```python
from build123d import *

# Parameters (mm, degrees)
BOSS_EXTRUDE1_DEPTH = 14
CUT_EXTRUDE1_DEPTH  = 17
CUT_EXTRUDE3_DEPTH  = 10
CUT_EXTRUDE5_DEPTH  = 28.00000000000001
BOSS_EXTRUDE2_START = 10
SKETCH7_R           = 2.599999999999999
BOSS_EXTRUDE2_DEPTH = 4
BOSS_EXTRUDE3_DEPTH = 24.000000000000014
CUT_EXTRUDE6_DEPTH  = 24.000000000000014
FILLET3_R           = 10.371224
SKETCH11_R          = 2.0000000000000036
BOSS_EXTRUDE4_DEPTH = 4.0000000000000036
SKETCH12_R          = 5.999999999999998
CUT_EXTRUDE7_DEPTH  = 2
CUT_EXTRUDE8_START  = -2
SKETCH13_R          = 6.000000000000001
CUT_EXTRUDE8_DEPTH  = 2


with BuildPart() as part:
    # Sketch1 → Boss-Extrude1 (new body)
    with BuildSketch(Plane.XY):
        with BuildLine():
            Line((-36.38946679579018, 35.15986129833476), (18.20052051694879, -13.03747639081095))
            Line((18.20052051694879, -13.03747639081095), (35.77692020217122, -13.037476390810937))
            ThreePointArc((35.77692020217122, -13.037476390810937), (35.15777812721451, -10.159169225075718), (33.40987673348322, -7.79002807961883))
            Line((33.40987673348322, -7.79002807961883), (-19.19377778956647, 51.90227090989418))
            ThreePointArc((-19.19377778956647, 51.90227090989418), (-36.16282709845803, 52.12891060722632), (-36.38946679579018, 35.15986129833476))
        make_face()
    extrude(amount=BOSS_EXTRUDE1_DEPTH)

    # Sketch2 → Cut-Extrude1 (cut)
    with BuildSketch(Plane.XY.offset(14)):
        with BuildLine():
            ThreePointArc((-26.066464510259447, 45.48286358386564), (-29.74341977242946, 45.48286358386556), (-29.74341977242945, 41.80590832169555))
            Line((-29.74341977242943, 41.80590832169553), (-26.066464510259397, 45.48286358386558))
        make_face()
        with BuildLine():
            Line((-26.066464510259397, 45.48286358386558), (-29.74341977242943, 41.80590832169553))
            ThreePointArc((-29.74341977242945, 41.805908321695554), (-26.90996521719519, 41.24229916825121), (-25.304942141344416, 43.64438595278056))
            ThreePointArc((-25.304942141344416, 43.64438595278056), (-25.502855356815083, 44.63936287692983), (-26.066464510259447, 45.48286358386564))
        make_face()
    extrude(amount=-CUT_EXTRUDE1_DEPTH, mode=Mode.SUBTRACT)

    # Sketch3 → Cut-Extrude3 (cut)
    with BuildSketch(Plane(origin=(0, 0, 0), x_dir=(-1, 0, 0), z_dir=(0, 0, -1))):
        Polygon((9.244950076252596, 40.61278154184911), (25.60190789451236, 23.944622093291866), (43.70935849975749, 23.944622093291866), (43.70935849975749, 56.22709716223903), (9.244950076252595, 56.22709716223903), align=None)
    extrude(amount=-CUT_EXTRUDE3_DEPTH, mode=Mode.SUBTRACT)

    # Sketch4 → Cut-Extrude5 (cut)
    with BuildSketch(Plane(origin=(1.5041731974177077, 1.7036790764832412, 0), x_dir=(0.7496354730351515, -0.6618509330410925, 0), z_dir=(-0.6618509330410925, -0.7496354730351515, 0))):
        with BuildLine():
            Line((8.092649067523661, 8), (43.108918661974144, 8))
            Line((43.108918661974144, 8), (43.108918661974144, 14))
            Line((43.108918661974144, 14), (-35.75655339767276, 14))
            add(Edge.make_bspline(
                [(8.092649067523661, 8), (-13.064100153172822, 13.584073422401662), (-35.75655339767276, 14)],
                knots=[0, 0, 0, 1, 1, 1], degree=2))
        make_face()
    extrude(amount=-CUT_EXTRUDE5_DEPTH, mode=Mode.SUBTRACT)



with BuildPart() as body_2:
    # Sketch7 → Boss-Extrude2 (new body)
    with BuildSketch(Plane(origin=(0, 0, 10), x_dir=(-1, 0, 0), z_dir=(0, 0, -1)).offset(BOSS_EXTRUDE2_START)):
        with BuildLine():
            Line((9.244950076252595, 40.61278154184911), (24.71284152511152, 24.85060352151197))
            Line((24.71284152511152, 24.85060352151197), (35.272794661727836, 34.17395478721706))
            Line((35.272794661727836, 34.17395478721706), (36.38946679579018, 35.15986129833476))
            ThreePointArc((36.38946679579018, 35.15986129833476), (36.27690366691708, 52.016347478352856), (19.420417486898984, 52.12891060722668))
            ThreePointArc((19.420417486898984, 52.128910607226686), (19.259089791001077, 51.96445532507904), (19.10094915036315, 51.79693307859034))
            Line((19.10094915036315, 51.79693307859034), (18.710021655268264, 51.3533258590539))
            Line((18.710021655268264, 51.3533258590539), (9.244950076252596, 40.61278154184911))
        make_face()
        with Locations(Location((27.904942141344414, 43.64438595278056, 0), (0, 0, 180))):
            Circle(SKETCH7_R, mode=Mode.SUBTRACT)
    extrude(amount=BOSS_EXTRUDE2_DEPTH)


with BuildPart() as part_1:
    add(part.part)

    add(body_2.part)  # Boss-Extrude3 merges body 2
    # Sketch9 → Boss-Extrude3 (add)
    with BuildSketch(Plane(origin=(14.941459139681696, 13.167114819822281, 0), x_dir=(0, 0, -1), z_dir=(0.7502493779859964, 0.6611549522098625, 0))):
        with BuildLine():
            Line((0, 36.582058615900806), (0, -5.650867010397978))
            add(Edge.make_bspline(
                [(0, -5.650867010397978), (3.8818367436513204, 15.308651069653255), (4, 36.582058615900806)],
                knots=[0, 0, 0, 1, 1, 1], degree=2))
            Line((4, 36.582058615900806), (0, 36.582058615900806))
        make_face()
    extrude(amount=-BOSS_EXTRUDE3_DEPTH)

    # Sketch10 → Cut-Extrude6 (cut)
    with BuildSketch(Plane.XY):
        Polygon((-25.92087579699025, 25.91717339280068), (6.581343150758677, -2.7789391982650153), (-1.9207549102098282, -11.21281031813962), (-35.1442259060093, 19.61838673287275), align=None)
    extrude(amount=-CUT_EXTRUDE6_DEPTH, mode=Mode.SUBTRACT)

    # Fillet3
    fillet3_edges = [part_1.edges().sort_by_distance(p)[0] for p in [
        (-24.712841525111525, 24.85060352151197, 5),
        (-9.244950076252596, 40.61278154184911, 5),
    ]]
    fillet(fillet3_edges, radius=FILLET3_R - 0.0001)  # a hair under: the kernel refuses the full size

    # Sketch11 → Boss-Extrude4 (add)
    with BuildSketch(Plane.XY.offset(14)):
        with BuildLine():
            Line((-56.27002242528391, 53.500762526462196), (-36.38946679579018, 35.15986129833476))
            Line((-36.38946679579018, 35.15986129833476), (-31.30885180689802, 50.34187338631568))
            Line((-31.30885180689802, 50.34187338631568), (-18.71002165526834, 51.353325859054))
            Line((-18.71002165526834, 51.353325859054), (-40.42419503361445, 70.87498928012118))
            ThreePointArc((-40.42419503361445, 70.87498928012118), (-57.13470265149496, 73.54200286861439), (-59.89717634802535, 56.84701064326646))
            Line((-59.89717634802535, 56.84701064326646), (-56.27002242528391, 53.500762526462196))
        make_face()
        with Locations((-50.120598780049356, 63.8053531942874)):
            Circle(SKETCH11_R, mode=Mode.SUBTRACT)
    extrude(amount=-BOSS_EXTRUDE4_DEPTH)

    # Sketch12 → Cut-Extrude7 (cut)
    with BuildSketch(Plane(origin=(0, 0, -4), x_dir=(-1, 0, 0), z_dir=(0, 0, -1))):
        with Locations((27.904942141344414, 43.64438595278056)):
            Circle(SKETCH12_R)
    extrude(amount=-CUT_EXTRUDE7_DEPTH, mode=Mode.SUBTRACT)

    # Sketch13 → Cut-Extrude8 (cut)
    with BuildSketch(Plane.XY.offset(14).offset(CUT_EXTRUDE8_START)):
        with Locations(Location((-27.904942141344414, 43.64438595278056, 0), (0, 0, 180))):
            Circle(SKETCH13_R)
    extrude(amount=CUT_EXTRUDE8_DEPTH, mode=Mode.SUBTRACT)


solid = part_1.part
```
Can you work these out from the model? Positions are in its coordinate system, mm. A direction names the side the tool comes from. Coordinates: 2 decimals unless noted, no trailing zeros. Order: outer loops, then holes, each group sorted by start corner. A loop starts at its lowest first (then second) coordinate and runs counter-clockwise, first axis right, second up. Notation, with made-up numbers: (47.25, 89.25) -> (81.25, 89.25) arc R30 cw to (81.25, 112.25) -> close; hole circle Ø2 at (61, 51.25). An arc over 180 degrees is marked (long way). Write each question's results on one line, items separated by ' | '.
Item 1: I want a section at C-C, the plane y = -5. Write out the boundary of the cut face in (x, z).
Results are:
outline: (9.1, 0) -> (30.95, 0) -> (30.95, 8) -> (9.1, 8) -> close
Item 2: Which directions (+Z, -Z, +X, -X, +Y, -Y) give clear straight access to the entire face, cutting with the end or side of a thin tool? Please do faces 1 (the face through (-29, 41, -2)), 2 (the face through (-9.49, 35.76, 5.07)), 3 (the face through (-29.2, 46.2, 12)), 4 (the face through (21, -4, 0)), 5 (the face through (-20.013, 24.901, 4.93)).
Results are:
face 1: -Z | face 2: +Y | face 3: +Z | face 4: -Z, +X, -Y | face 5: -X
Item 3: If I drill on line 1 along Z through (x, y) = (-23.5, 37); line 2 along Y through (x, z) = (-13, -2.25); line 3 along Y through (x, z) = (30.5, 6.25), over which ranges is the centre line in solid material (lowest first)?
Results are:
line 1: -4 to 0, 10 to 14 | line 2: 14.51 to 44.87 | line 3: -13.04 to -4.49
Item 4: I'm going to push flat-ended pins straight in: pin 1 Ø4 at (x, y) = (-27.9, 43.64) entering from -Z; pin 2 Ø7 at (x, y) = (-27.9, 43.64) entering from +Z; pin 3 Ø8 at (x, z) = (-12.5, -1.5) entering from -Y; pin 4 Ø17.5 at (x, y) = (14, -1.5) entering from -Z. Where does each tip first touch, or does it pass through?
Results are:
pin 1: through | pin 2: z = 12 | pin 3: y = 10.54 | pin 4: z = -0.71
Item 5: If we mould it in two halves opening along Y, with no side actions, what happens to faces 6 (the face through (-36.46, 51.83, -1.97)), 7 (the face through (35.175, -10.197, 3.944)), 8 (the face through (-26.51, 41.45, -0.99))? For each: +Y half, -Y half, draft (parallel to the pull), parting line (faces both ways), or undercut.
Results are:
face 6: parting line | face 7: +Y half | face 8: undercut
Item 6: I want a section at B-B, the plane x = -27. Write out the boundary of the cut face in (y, z), then the cut area to 3 significant figures.
Results are:
outline: (26.87, -4) -> (37.71, -4) -> (37.71, -2) -> (41.21, -2) -> (41.21, 0) -> (26.87, 0) -> close; (26.87, 10) -> (41.21, 10) -> (41.21, 12) -> (37.71, 12) -> (37.71, 14) -> (26.87, 14) -> close; (46.08, -2) -> (49.58, -2) -> (49.58, -4) -> (55.5, -4) -> (55.5, 0) -> (46.08, 0) -> close; (46.08, 10) -> (58.81, 10) -> (58.81, 14) -> (49.58, 14) -> (49.58, 12) -> (46.08, 12) -> close | area: 175 mm²
